For this review, take the finished solid that the model builds, in its own axes (mm). Round coordinates to 2 decimals unless told otherwise and drop trailing zeros. Write each loop counter-clockwise with the first axis right and the second up, starting at its lowest first coordinate (ties: lowest second). Pieces come first, ordered by that corner, then holes. Notation, with made-up numbers: (14.25, 32.5) -> (40.25, 32.5) arc R21 ccw to (40.25, 71.5) -> close; hole circle Ø5 at (28, -5.5). An arc over 180 degrees is marked (long way). Answer in a Markdown table with one row per item.
Autodesk Fusion 360 part; units mm, degrees
sketch "main_driver" plane through (0, 0, 0) normal (1, 0, 0) x (0, 1, 0)
  line L0 (150, 45.3) -> (154.0703, 47.65)
  line L1 (154.0703, 47.65) -> (154.0703, 52.35)
  line L2 (154.0703, 52.35) -> (150, 54.7)
  line L3 (150, 54.7) -> (145.9297, 52.35)
  line L4 (145.9297, 52.35) -> (145.9297, 47.65)
  line L5 (145.9297, 47.65) -> (150, 45.3)
  point P0 (150, 50)
  dimension "d1" = 4.7
extrude "Extrude1" add sketch "main_driver" against normal blind 150
fillet "Fillet1" radius 0.75 12 edges at (-150, 147.9648, 53.525) (-150, 152.0352, 53.525) (-150, 154.0703, 50) (-150, 152.0352, 46.475) (-150, 147.9648, 46.475) (-150, 145.9297, 50) (0, 152.0352, 53.525) (0, 147.9648, 53.525) (0, 145.9297, 50) (0, 147.9648, 46.475) (0, 152.0352, 46.475) (0, 154.0703, 50)
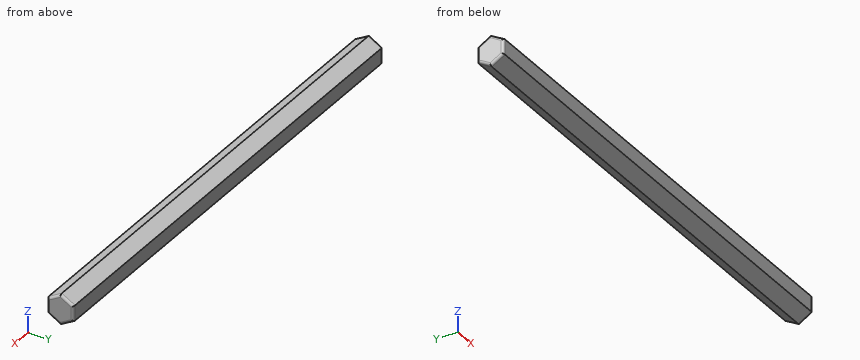
1) For line 1 (Z direction, x = -123, y = 148.5); line 2 (X direction, y = 153, z = 47.5); line 3 (Z direction, x = -26, y = 150.5), list the stretches that pass through material, from the lowest coordinate up. Write a range as [from, to].
Solved:
| item | result |
|---|---|
| line 1 | [46.17, 53.83] |
| line 2 | [-149.92, -0.08] |
| line 3 | [45.59, 54.41] |
2) Clearance check with flat-ended pins moving along their axes: pin 1 Ø2 at (x, y) = (-127, 151.5) entering from +Z; pin 2 Ø2 at (x, y) = (-40.5, 147.5) entering from -Z. State where each tip first meets the part, or that it passes through.
Solved:
| item | result |
|---|---|
| pin 1 | z = 54.41 |
| pin 2 | z = 46.17 |
3) Consider section A-A on x = -32. State the section outline as (y, z) points, then the cut area to 3 significant figures.
Solved:
| item | result |
|---|---|
| outline | (145.93, 47.65) -> (150, 45.3) -> (154.07, 47.65) -> (154.07, 52.35) -> (150, 54.7) -> (145.93, 52.35) -> close |
| area | 57.4 mm² |
